from build123d import *

# Parameters (mm, degrees)
CROQUIS5_R              = 7.9375
CORTAR_EXTRUIR3_DEPTH   = 18
CROQUIS9_R              = 3.175
CORTAR_EXTRUIR5_DEPTH   = 18
CROQUIS10_R             = 4.765
CORTAR_EXTRUIR6_DEPTH   = 35
CROQUIS11_R             = 35
SALIENTE_EXTRUIR1_DEPTH = 14.24


with BuildPart() as part:
    # Croquis1 → Revolución3 (revolve)
    with BuildSketch(Plane.XY, mode=Mode.PRIVATE) as revoluci_n3_sk:
        with BuildLine():
            Line((0, 43.044568245), (30, 43.044568245))
            Line((30, 43.044568245), (30, 20.044568245))
            Line((30, 20.044568245), (12.985796912, 20.044568245))
            Line((12.985796912, 20.044568245), (12.985796912, 10.406207601))
            ThreePointArc((12.985796912, 10.406207601), (13.175212613, 9.391052882), (13.717969076, 8.512512712))
            Line((13.717969076, 8.512512712), (32.309744815, 5.485961945))
            ThreePointArc((32.309744815, 5.485961945), (33.884795273, 4.831882369), (35, 3.541563627))
            Line((35, 3.541563627), (35, -0.490098714))
            Line((35, -0.490098714), (13.468735488, -0.490098714))
            Line((13.468735488, -0.490098714), (13.468735488, -18.538757946))
            Line((13.468735488, -18.538757946), (31.979226627, -20.513196287))
            ThreePointArc((31.979226627, -20.513196287), (33.927671218, -21.380602851), (35, -23.224224681))
            Line((35, -23.224224681), (35, -35.501069654))
            Line((35, -35.501069654), (24.334695592, -35.501069654))
            Line((24.334695592, -35.501069654), (24.334695592, -43.520130292))
            Line((24.334695592, -43.520130292), (34.538342083, -43.520130292))
            Line((34.538342083, -43.520130292), (34.538342083, -52.477142798))
            Line((34.538342083, -52.477142798), (24.334695592, -52.477142798))
            Line((24.334695592, -52.477142798), (24.334695592, -58.946096275))
            Line((24.334695592, -58.946096275), (34.538342083, -58.946096275))
            Line((34.538342083, -58.946096275), (34.538342083, -64.917437946))
            Line((34.538342083, -64.917437946), (24.334695592, -64.917437946))
            Line((24.334695592, -64.917437946), (24.334695592, -72.132809132))
            Line((24.334695592, -72.132809132), (34.538342083, -72.132809132))
            Line((34.538342083, -72.132809132), (34.538342083, -77.357733094))
            Line((34.538342083, -77.357733094), (24.334695592, -77.357733094))
            Line((24.334695592, -77.357733094), (24.334695592, -104.221668074))
            Line((24.334695592, -104.221668074), (34.538342083, -104.221668074))
            ThreePointArc((34.538342083, -104.221668074), (34.864783527, -104.356884547), (35, -104.683325991))
            Line((35, -104.683325991), (35, -120.950877143))
            ThreePointArc((35, -120.950877143), (34.933442046, -121.487214162), (34.737806004, -121.991013624))
            Line((34.737806004, -121.991013624), (0, -121.955431755))
            Line((0, -121.955431755), (0, 43.044568245))
        make_face()
    revolve(revoluci_n3_sk.sketch.rotate(Axis((0, 43.044568245, 0), (0, -1, 0)), 180), axis=Axis((0, 43.044568245, 0), (0, -1, 0)))

    # Croquis5 → Cortar-Extruir3 (cut)
    with BuildSketch(Plane(origin=(0, -104.221668074, 0), x_dir=(1, 0, 0), z_dir=(0, 1, 0))):
        with Locations(Location((0.097949209, 0, 0), (0, 0, 270))):
            Circle(CROQUIS5_R)
    extrude(amount=-CORTAR_EXTRUIR3_DEPTH, mode=Mode.SUBTRACT)

    # Croquis9 → Cortar-Extruir5 (cut)
    with BuildSketch(Plane(origin=(0, 43.044568245, 0), x_dir=(1, 0, 0), z_dir=(0, 1, 0))):
        with Locations(Location((0, 23, 0), (0, 0, 180))):
            Circle(CROQUIS9_R)
        with Locations(Location((0, -23, 0), (0, 0, 180))):
            Circle(CROQUIS9_R)
    extrude(amount=-CORTAR_EXTRUIR5_DEPTH, mode=Mode.SUBTRACT)

    # Croquis10 → Cortar-Extruir6 (cut)
    with BuildSketch(Plane(origin=(0, 43.044568245, 0), x_dir=(1, 0, 0), z_dir=(0, 1, 0))):
        with Locations(Location((0, 0, 0), (0, 0, 180))):
            Circle(CROQUIS10_R)
    extrude(amount=-CORTAR_EXTRUIR6_DEPTH, mode=Mode.SUBTRACT)

    # Croquis11 → Saliente-Extruir1 (add)
    with BuildSketch(Plane(origin=(0, -104.221668074, 0), x_dir=(1, 0, 0), z_dir=(0, 1, 0))):
        with Locations(Location((0, 0, 0), (0, 0, 180))):
            Circle(CROQUIS11_R)
    extrude(amount=SALIENTE_EXTRUIR1_DEPTH)


solid = part.part
For this review, take the finished solid that the model builds, in its own axes (mm). A direction names the side the tool comes from. Give positions to 0.01 mm unless a question says otherwise; leave off trailing zeros. Order: outer loops, then holes, each group sorted by start corner. A loop starts at its lowest first (then second) coordinate and runs counter-clockwise, first axis right, second up. Notation, with made-up numbers: (88.5, -26.5) -> (142.5, -26.5) arc R18 cw to (142.5, 1.5) -> close; hole circle Ø11 at (-15, 73.25). An arc over 180 degrees is marked (long way). Write item = value, one per line.
1) We need section B-B, the plane x = -16. Count the separate pieces of the cut face and the enclosed holes in it, and give its area (3 significant figures).
Findings:
separate_pieces = 3
enclosed_holes = 0
area = 7,100 mm^2
2) Draft analysis for pull direction Y (two halves, no side actions). For faces 3 (the face through (-6.749, -18.662, 12.976)), 4 (the face through (0, 25.045, -23)), 5 (the face through (0.41, 34.17, -19.85)), state which applies: pulls with the +Y half, pulls with the -Y half, needs draft (parallel to the pull), parting line crosses it, or undercut.
Findings:
face_3 = undercut
face_4 = pulls with the +Y half
face_5 = needs draft
3) Insertion check: pin 1 (10 mm diameter, centred on x = -14, y = -31, fed in from -Z); pin 2 (18.5 mm diameter, centred on x = 0.1, z = 0, fed in from -Y) (3 decimals); pin 3 (5 mm diameter, centred on x = -2, z = 3.5, fed in from -Y). Each pin has a flat end and moves straight along its axis. Give the tip position at first contact, or say it passes through.
Findings:
pin_1 = -33.82
pin_2 = -121.965
pin_3 = -104.22
4) We need section A-A, the plane y = -96.5. Give the boundary of the cut face in (x, z), and give its area (3 significant figures).
Findings:
outline = circle Ø70 at (0, 0)
area = 3,850 mm^2
5) For faces 1 (the face through (-6, 20.045, 13)), 2 (the face through (0.69, 34.17, 19.9)), list the 3-axis set-ups (+Z, -Z, +X, -X, +Y, -Y) from which the entire face can be reached by the end or side of a thin tool; tool diameter is ignored.
Findings:
face_1 = none
face_2 = +Y
6) To check wall thickness, follow L1, parallel to Z at x = 0, y = 36.25 (3 decimals); L2, parallel to Z at x = 0, y = 16 (3 decimals); L3, parallel to Y at x = -30, z = 3. State the ranges of each line that lie inside material, in increasing order. Write a range as from..to.
Findings:
L1 = -30..-26.175, -19.825..-4.765, 4.765..19.825, 26.175..30
L2 = -12.986..-4.765, 4.765..12.986
L3 = -121.99..-89.98, -77.36..-72.13, -64.92..-58.95, -52.48..-43.52, -35.5..-20.32, -0.49..5.84
